The model under review builds one solid part; all positions refer to its coordinate system, in mm. Face numbers are marked on the shaded views. A direction names the side the tool comes from. Give positions to 0.01 mm unless a question says otherwise; leave off trailing zeros. Order: outer loops, then holes, each group sorted by start corner. A loop starts at its lowest first (then second) coordinate and runs counter-clockwise, first axis right, second up.
```python
from build123d import *

# Parameters (mm, degrees)
F0_W      = 43
F0_H      = 46
F1_DEPTH  = 25
F2_R      = 3
F3_T      = -2
F4_R      = 8
F5_DEPTH  = 2
F6_R      = 3.1
F7_DEPTH  = 2
F8_R      = 1.75
F9_DEPTH  = 7.5
F11_R     = 0.9
F12_DEPTH = 7
F15_DEPTH = 3
F16_R     = 2.4
F17_DEPTH = 5


with BuildPart() as f1:
    # F0 (on Top) → F1 (new body)
    with BuildSketch(Plane.XY):
        Rectangle(F0_W, F0_H)
    extrude(amount=F1_DEPTH)

    # F2
    f2_edges = [f1.edges().sort_by_distance(p)[0] for p in [
        (21.5, 0, 0),
        (0, -23, 0),
        (0, 23, 0),
        (-21.5, 0, 0),
        (21.5, 23, 12.5),
        (21.5, -23, 12.5),
        (-21.5, -23, 12.5),
        (-21.5, 23, 12.5),
    ]]
    fillet(f2_edges, radius=F2_R)

    # F3
    f3_openings = [f1.faces().sort_by_distance(p)[0] for p in [
        (0, 0, 25),
    ]]
    offset(amount=F3_T, openings=f3_openings)

    # F4 (on face) → F5 (cut, through all)
    with BuildSketch(Plane.XY.offset(2)):
        Circle(F4_R)
    extrude(amount=-F5_DEPTH, mode=Mode.SUBTRACT)

    # F6 (on face) → F7 (cut, through all)
    with BuildSketch(Plane.YZ.offset(21.5)):
        with Locations((-9, 16)):
            Circle(F6_R)
    extrude(amount=-F7_DEPTH, mode=Mode.SUBTRACT)

    # F8 (on face) → F9 (join)
    with BuildSketch(Plane.XY.offset(2)):
        with Locations((17, 17)):
            Circle(F8_R)
        with Locations((17, -17)):
            Circle(F8_R)
        with Locations((-17, -17)):
            Circle(F8_R)
    extrude(amount=F9_DEPTH)

    # F11 (on offset) → F12 (cut)
    with BuildSketch(Plane.XY.offset(9.5)):
        with Locations((17, 17)):
            Circle(F11_R)
        with Locations((17, -17)):
            Circle(F11_R)
        with Locations((-17, -17)):
            Circle(F11_R)
    extrude(amount=-F12_DEPTH, mode=Mode.SUBTRACT)

    # F14 (on offset) → F15 (cut)
    with BuildSketch(Plane.XY.offset(25)):
        with BuildLine():
            Line((-18.5, -22), (18.5, -22))
            ThreePointArc((18.5, -22), (19.9142135624, -21.4142135624), (20.5, -20))
            Line((20.5, -20), (20.5, 20))
            ThreePointArc((20.5, 20), (19.9142135624, 21.4142135624), (18.5, 22))
            Line((18.5, 22), (-18.5, 22))
            ThreePointArc((-18.5, 22), (-19.9142135624, 21.4142135624), (-20.5, 20))
            Line((-20.5, 20), (-20.5, -20))
            ThreePointArc((-20.5, -20), (-19.9142135624, -21.4142135624), (-18.5, -22))
        make_face()
    extrude(amount=-F15_DEPTH, mode=Mode.SUBTRACT)

    # F16 (on face) → F17 (join)
    with BuildSketch(Plane.XY.offset(2)):
        with Locations((17, 17)):
            Circle(F16_R)
        with Locations((17, -17)):
            Circle(F16_R)
        with Locations((-17, -17)):
            Circle(F16_R)
    extrude(amount=F17_DEPTH)


solid = f1.part
```
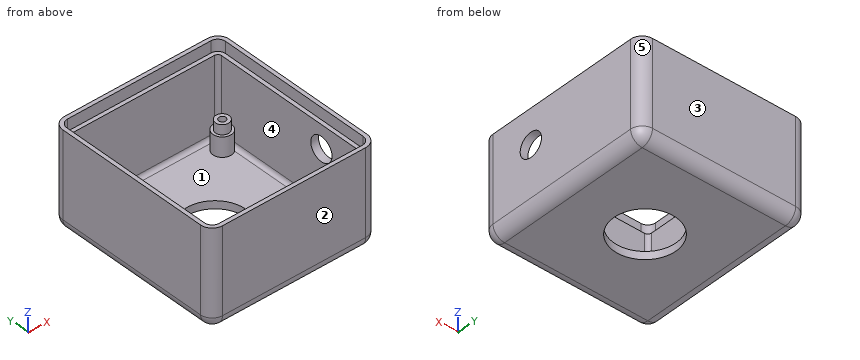
Item 1: Take a section at B-B (x = 0). Give the boundary of the cut face in (y, z).
Values found:
outline: (-23, 3) arc R3 ccw to (-20, 0) - (-8, 0) - (-8, 2) - (-20, 2) arc R1 cw to (-21, 3) - (-21, 22) - (-22, 22) - (-22, 25) - (-23, 25) - close; (8, 0) - (20, 0) arc R3 ccw to (23, 3) - (23, 25) - (22, 25) - (22, 22) - (21, 22) - (21, 3) arc R1 cw to (20, 2) - (8, 2) - close
Item 2: For line 1 (Y direction, x = 17, z = 8); line 2 (Y direction, x = 13, z = 3.75); line 3 (X direction, y = 5, z = 6.25), list the stretches that pass through material, from the lowest coordinate up.
Values found:
line 1: y = -23 to -21, -18.75 to -17.9, -16.1 to -15.25, 15.25 to 16.1, 17.9 to 18.75, 21 to 23
line 2: y = -23 to -21, 21 to 23
line 3: x = -21.5 to -19.5, 19.5 to 21.5
Item 3: Take a section at A-A (z = 5.5). Give the boundary of the cut face in (x, y).
Values found:
outline: (-21.5, -20) arc R3 ccw to (-18.5, -23) - (18.5, -23) arc R3 ccw to (21.5, -20) - (21.5, 20) arc R3 ccw to (18.5, 23) - (-18.5, 23) arc R3 ccw to (-21.5, 20) - close; circle Ø4.8 at (-17, -17); circle Ø4.8 at (17, -17); circle Ø4.8 at (17, 17); hole (-19.5, -20) arc R1 ccw to (-18.5, -21) - (18.5, -21) arc R1 ccw to (19.5, -20) - (19.5, 20) arc R1 ccw to (18.5, 21) - (-18.5, 21) arc R1 ccw to (-19.5, 20) - close
Item 4: Take a section at D-D (x = -17). Give the boundary of the cut face in (y, z).
Values found:
outline: (-23, 3) arc R3 ccw to (-20, 0) - (20, 0) arc R3 ccw to (23, 3) - (23, 25) - (22, 25) - (22, 22) - (21, 22) - (21, 3) arc R1 cw to (20, 2) - (-14.6, 2) - (-14.6, 7) - (-15.25, 7) - (-15.25, 9.5) - (-16.1, 9.5) - (-16.1, 7) - (-17.9, 7) - (-17.9, 9.5) - (-18.75, 9.5) - (-18.75, 7) - (-19.4, 7) - (-19.4, 2) - (-20, 2) arc R1 cw to (-21, 3) - (-21, 22) - (-22, 22) - (-22, 25) - (-23, 25) - close
Item 5: Draft analysis for pull direction Y (two halves, no side actions). For the marked faces 1, 2 and 3, state which applies: released by +Y, released by -Y, zero draft, split by the parting line, or undercut.
Values found:
face 1: undercut
face 2: released by -Y
face 3: released by +Y
Item 6: Take a section at C-C (y = 0). Give the boundary of the cut face in (x, z), and give its area (3 significant figures).
Values found:
outline: (-21.5, 3) arc R3 ccw to (-18.5, 0) - (-8, 0) - (-8, 2) - (-18.5, 2) arc R1 cw to (-19.5, 3) - (-19.5, 22) - (-20.5, 22) - (-20.5, 25) - (-21.5, 25) - close; (8, 0) - (18.5, 0) arc R3 ccw to (21.5, 3) - (21.5, 25) - (20.5, 25) - (20.5, 22) - (19.5, 22) - (19.5, 3) arc R1 cw to (18.5, 2) - (8, 2) - close
area: 137 mm2
Item 7: Clearance check with flat-ended pins moving along their axes: pin 1 Ø3 at (x, y) = (17, -17) entering from +Z; pin 2 Ø3 at (x, y) = (9.5, -9.5) entering from +Z; pin 3 Ø1.4 at (x, y) = (17, 17) entering from +Z; pin 4 Ø13 at (x, y) = (0, 0) entering from +Z. State where each tip first meets the part, or that it passes through.
Values found:
pin 1: stops at z = 9.5
pin 2: stops at z = 2
pin 3: stops at z = 7
pin 4: passes through
Item 8: For the marked faces 4 and 5, list the 3-axis set-ups (+Z, -Z, +X, -X, +Y, -Y) from which the entire face can be reached by the end or side of a thin tool; tool diameter is ignored.
Values found:
face 4: +Z
face 5: +Z, -Z, +X, +Y
